Autodesk Inventor part; units mm, degrees
ref_plane "bolt_XY" through (0, 0, 0) normal (1, 0, 0) x (0, 0, -1)
ref_plane "bolt_YZ" through (0, 0, 0) normal (0, 0, -1) x (0, 1, 0)
ref_plane "bolt_ZX" through (0, 0, 0) normal (0, 1, 0) x (1, 0, 0)
sketch "Sketch_1" plane through (0, 0, 0) normal (0, 0, 1) x (1, 0, 0)
  line L0 (6, 0) -> (-4, 0)
  line L1 (-4, 0) -> (-4, 3.5)
  line L2 (-4, 3.5) -> (0, 3.5)
  line L3 (0, 3.5) -> (0, 2)
  line L4 (0, 2) -> (5.5705, 2)
  line L5 (5.5705, 2) -> (6, 1.5705)
  line L6 (6, 1.5705) -> (6, 0)
  line L7 (6, 0) -> (-4, 0)
revolve "Revolution1" add sketch "Sketch_1" angle 360 about axis through (6, 0, 0) along (1, 0, 0)
thread "Thread1"
sketch "Sketch_4" plane through (0, 0, 0) normal (0, 0, 1) x (1, 0, 0)
  line L0 (-1.5981, 0) -> (-4, 0)
  line L1 (-4, 0) -> (-4, 1.5)
  line L2 (-4, 1.5) -> (-2, 1.5)
  line L3 (-2, 1.5) -> (-1.5981, 0)
  line L4 (-1.5981, 0) -> (-4, 0)
revolve "Revolution2" cut sketch "Sketch_4" angle 360 about axis through (-1.5981, 0, 0) along (1, 0, 0)
sketch "Sketch_3" plane through (-4, 0, 0) normal (1, 0, 0) x (0, 0, -1)
  line L0 (-1.5, 0.866) -> (-1.5, -0.866)
  line L1 (-1.5, -0.866) -> (0, -1.7321)
  line L2 (0, -1.7321) -> (1.5, -0.866)
  line L3 (1.5, -0.866) -> (1.5, 0.866)
  line L4 (1.5, 0.866) -> (0, 1.7321)
  line L5 (0, 1.7321) -> (-1.5, 0.866)
extrude "Extrusion1" cut sketch "Sketch_3" along normal blind 2
ref_plane "bolt_XY" through (0, 0, 0) normal (1, 0, 0) x (0, 0, -1)
ref_plane "bolt_YZ" through (0, 0, 0) normal (0, 0, -1) x (0, 1, 0)
ref_plane "bolt_ZX" through (0, 0, 0) normal (0, 1, 0) x (1, 0, 0)
ref_plane "nut_XY" through (6, 0, 0) normal (1, 0, 0) x (0, 0, -1)
ref_plane "nut_YZ" through (6, 0, 0) normal (0, 0, -1) x (0, 1, 0)
ref_plane "nut_ZX" through (6, 0, 0) normal (0, 1, 0) x (1, 0, 0)
properties part number "CBM4-6" material "MISUMI"
For this review, take the finished solid that the model builds, in its own axes (mm). A direction names the side the tool comes from. Round coordinates to 2 decimals unless told otherwise and drop trailing zeros. Write each loop counter-clockwise with the first axis right and the second up, starting at its lowest first coordinate (ties: lowest second). Pieces come first, ordered by that corner, then holes. Notation, with made-up numbers: (64.25, 88) - (81.25, 88) arc R14 ccw to (81.25, 98) - close; hole circle Ø11 at (9, 48). An arc over 180 degrees is marked (long way). Use CSV: the item, a comma, the result in double quotes.
1) Wall thickness on line 1 along X through (y, z) = (-1.5, 0.25); line 2 along X through (y, z) = (-0.5, -2.25); line 3 along Y through (x, z) = (2.5, -1): over which ranges is each line inside the solid? List them lowest first. Write a range as from..to.
Conclusion:
line 1,"x = -2..6"
line 2,"x = -4..0"
line 3,"y = -1.73..1.73"
2) Add section B-B on y = 2.5. Write out the cut boundary in (x, z), and give its area (3 significant figures).
Conclusion:
outline,"(-4, -2.45) - (0, -2.45) - (0, 2.45) - (-4, 2.45) - close"
area,"19.6 mm^2"
3) For faces 4 (the flat face through (0, 2, -2)), 5 (the flat face through (6, 0, 0)), 6 (the flat face through (-3.014, 1.293, -0.76)), list the 3-axis set-ups (+Z, -Z, +X, -X, +Y, -Y) from which the entire face can be reached by the end or side of a thin tool; tool diameter is ignored.
Conclusion:
face 4,"+X"
face 5,"+Z, -Z, +X, +Y, -Y"
face 6,"-X"
4) Clearance check with flat-ended pins moving along their axes: pin 1 Ø0.9 at (y, z) = (-0.5, 0) entering from -X; pin 2 Ø1 at (x, z) = (-1.5, -1.5) entering from -Y; pin 3 Ø4 at (x, y) = (2.5, 1) entering from -Z. State where each tip first meets the part, or that it passes through.
Conclusion:
pin 1,"stops at x = -1.85"
pin 2,"stops at y = -3.35"
pin 3,"stops at z = -2"
5) Add section A-A on x = 4.5. Write out the cut boundary in (y, z).
Conclusion:
outline,"circle Ø4 at (0, 0)"
6) The part is to be moulded in two halves that separate along Y. For faces 1 (the flat face through (-3, 0, 1.5)), 2 (the flat face through (-4, 0, -2)), 3 (the cylindrical face through (3, 0, -2)), say which applies: pulls with the +Y half, pulls with the -Y half, needs draft (parallel to the pull), parting line crosses it, or undercut.
Conclusion:
face 1,"undercut"
face 2,"needs draft"
face 3,"parting line crosses it"
